Read the model definition and answer for the solid it produces. Units are mm, in the model's axes. Coordinates: 2 decimals unless noted, no trailing zeros. Write each loop counter-clockwise with the first axis right and the second up, starting at its lowest first coordinate (ties: lowest second). Pieces come first, ordered by that corner, then holes.
1) The part is cut by section B-B (y = 0). Determine the outline of the cut face in (x, z), then the cut area to 3 significant figures.
2) Determine the mould class of faces 1 (the face through (0, -2, 2)), 2 (the face through (2, 5, 0.8)), 3 (the face through (-1.08, -4.88, 2.42)), 4 (the face through (-2, 3, 3.95)) for opening direction X: +X half, -X half, draft (parallel to the pull), parting line (faces both ways), or undercut.
3) The part is cut by section A-A (z = 1.85). Determine the outline of the cut face in (x, y).
4) The part is cut by section C-C (x = 1). Determine the outline of the cut face in (y, z).
5) Each of these flat-tipped pins is pushed along its axis until it touches: pin 1 Ø1 at (x, z) = (4, 3) entering from -Y; pin 2 Ø1.5 at (y, z) = (4.5, 0.5) entering from -X. Where does it stop, or does it pass through?
6) The part is cut by section D-D (x = -2.75). Determine the outline of the cut face in (y, z).
7) Find the intervals of material crossed by line 1 (Z direction, x = -3.75, y = -4); line 2 (Z direction, x = 2.75, y = 2.5); line 3 (X direction, y = 3, z = 0.65), in increasing order.
from build123d import *

# Parameters (mm, degrees)
F2_R     = 4.2
F2_R_2   = 3
F3_DEPTH = 3
F4_R     = 4.15
F4_R_2   = 3.05
F5_DEPTH = 2.95


with BuildPart() as f1:
    # F0 (on Front) → F1 (revolve)
    with BuildSketch(Plane.XZ):
        Polygon((2, 4), (2, 0), (5.8, 0), (5.8, 0.8), (5, 0.8), (5, 4), align=None)
    revolve(axis=Axis((0, 0, 2), (0, 0, 1)))

    # F2 (on face) → F3 (cut)
    with BuildSketch(Plane.XY.offset(4)):
        Circle(F2_R)
        Circle(F2_R_2, mode=Mode.SUBTRACT)
    extrude(amount=-F3_DEPTH, mode=Mode.SUBTRACT)

    # F4 (on face) → F5 (join)
    with BuildSketch(Plane.XY.offset(1)):
        Circle(F4_R)
        Circle(F4_R_2, mode=Mode.SUBTRACT)
    extrude(amount=F5_DEPTH)


solid = f1.part
Reported:
1. outline: (-5.8, 0) - (-2, 0) - (-2, 4) - (-3, 4) - (-3, 1) - (-3.05, 1) - (-3.05, 3.95) - (-4.15, 3.95) - (-4.15, 1) - (-4.2, 1) - (-4.2, 4) - (-5, 4) - (-5, 0.8) - (-5.8, 0.8) - close; (2, 0) - (5.8, 0) - (5.8, 0.8) - (5, 0.8) - (5, 4) - (4.2, 4) - (4.2, 1) - (4.15, 1) - (4.15, 3.95) - (3.05, 3.95) - (3.05, 1) - (3, 1) - (3, 4) - (2, 4) - close
1. area: 24.6 mm2
2. face 1: undercut
2. face 2: draft
2. face 3: parting line
2. face 4: undercut
3. outline: circle Ø10 at (0, 0); circle Ø8.3 at (0, 0); circle Ø6 at (0, 0); hole circle Ø8.4 at (0, 0); hole circle Ø6.1 at (0, 0); hole circle Ø4 at (0, 0)
4. outline: (-5.71, 0) - (-1.73, 0) - (-1.73, 4) - (-2.83, 4) - (-2.83, 1) - (-2.88, 1) - (-2.88, 3.95) - (-4.03, 3.95) - (-4.03, 1) - (-4.08, 1) - (-4.08, 4) - (-4.9, 4) - (-4.9, 0.8) - (-5.71, 0.8) - close; (1.73, 0) - (5.71, 0) - (5.71, 0.8) - (4.9, 0.8) - (4.9, 4) - (4.08, 4) - (4.08, 1) - (4.03, 1) - (4.03, 3.95) - (2.88, 3.95) - (2.88, 1) - (2.83, 1) - (2.83, 4) - (1.73, 4) - close
5. pin 1: stops at y = -3.57
5. pin 2: stops at x = -4.42
6. outline: (-5.11, 0) - (5.11, 0) - (5.11, 0.8) - (4.18, 0.8) - (4.18, 4) - (3.17, 4) - (3.17, 1) - (3.11, 1) - (3.11, 3.95) - (1.32, 3.95) - (1.32, 1) - (1.2, 1) - (1.2, 4) - (-1.2, 4) - (-1.2, 1) - (-1.32, 1) - (-1.32, 3.95) - (-3.11, 3.95) - (-3.11, 1) - (-3.17, 1) - (-3.17, 4) - (-4.18, 4) - (-4.18, 0.8) - (-5.11, 0.8) - close
7. line 1: z = 0 to 0.8
7. line 2: z = 0 to 3.95
7. line 3: x = -4.96 to 4.96
